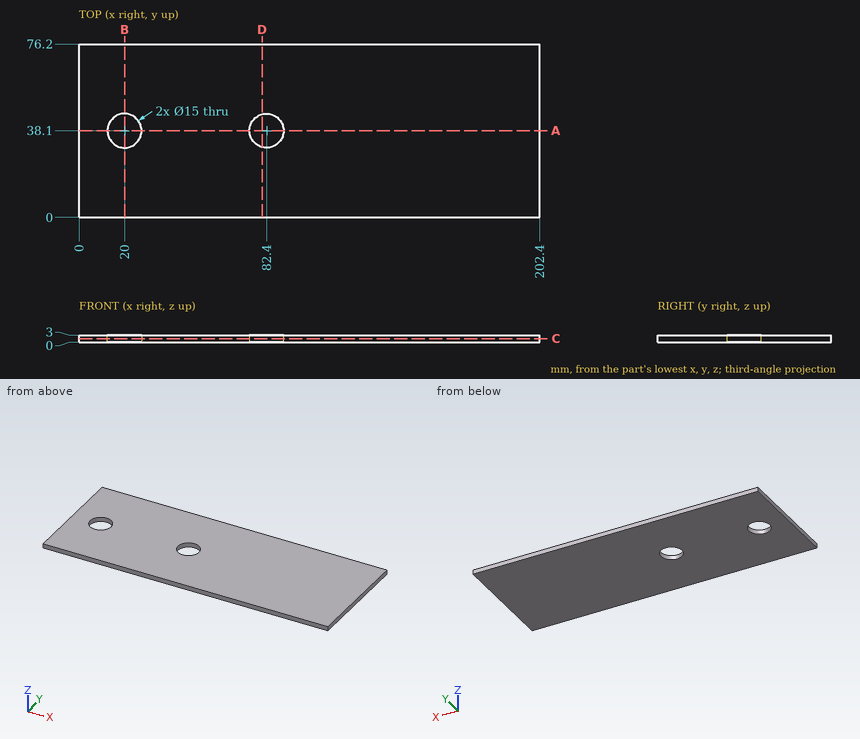
Design review of the part shown in the three views and the two pictorial views. Dimensions are in mm from the part's minimum x, y and z. Give positions to 0.01 mm unless a question says otherwise; leave off trailing zeros. Loops run counter-clockwise (first coordinate to the right, second up) from the corner with the lowest first, then second, coordinate; pieces in that order, holes last. Notation, with made-up numbers: (-28, -24) -> (-19, -24) arc R17 ccw to (-19, -10) -> close; hole circle Ø6 at (1, 27). An arc over 180 degrees is marked (long way). Write each question's results on one line, items separated by ' | '.
Q1. Take a section at C-C, the plane z = 1.6. Write out the cut boundary in (x, y), plus the area to 3 significant figures.
Reply:
outline: (0, 0) -> (202.4, 0) -> (202.4, 76.2) -> (0, 76.2) -> close; hole circle Ø15 at (20, 38.1); hole circle Ø15 at (82.4, 38.1) | area: 15,100 mm²
Q2. Wall thickness on L1, parallel to Y at x = 82.4, z = 1.8; L2, parallel to X at y = 44, z = 2.75; L3, parallel to Y at x = 18, z = 1.9: over which ranges is each line inside the solid? List them lowest first.
Reply:
L1: y = 0 to 30.6, 45.6 to 76.2 | L2: x = 0 to 15.37, 24.63 to 77.77, 87.03 to 202.4 | L3: y = 0 to 30.87, 45.33 to 76.2
Q3. Take a section at D-D, the plane x = 80.5. Write out the cut boundary in (y, z).
Reply:
outline: (0, 0) -> (30.84, 0) -> (30.84, 3) -> (0, 3) -> close; (45.36, 0) -> (76.2, 0) -> (76.2, 3) -> (45.36, 3) -> close
Q4. For pin 1 Ø9 at (x, y) = (82.4, 38.1) entering from +Z, flat-tipped, find the tip position at first contact; note if it passes through.
Reply:
pin 1: passes through
Q5. Take a section at A-A, the plane y = 38.1. Write out the cut boundary in (x, z), plus the area to 3 significant figures.
Reply:
outline: (0, 0) -> (12.5, 0) -> (12.5, 3) -> (0, 3) -> close; (27.5, 0) -> (74.9, 0) -> (74.9, 3) -> (27.5, 3) -> close; (89.9, 0) -> (202.4, 0) -> (202.4, 3) -> (89.9, 3) -> close | area: 517 mm²
Q6. Take a section at B-B, the plane x = 20. Write out the cut boundary in (y, z), plus the area to 3 significant figures.
Reply:
outline: (0, 0) -> (30.6, 0) -> (30.6, 3) -> (0, 3) -> close; (45.6, 0) -> (76.2, 0) -> (76.2, 3) -> (45.6, 3) -> close | area: 184 mm²
